Check sheet for the modelled part. Datum: model origin and axes. Units: mm. A direction names the side the tool comes from. Give positions to 0.01 mm unless a question says otherwise; leave off trailing zeros. Write each loop counter-clockwise with the first axis right and the second up, starting at its lowest first coordinate (ties: lowest second). Pieces come first, ordered by that corner, then holes. Notation, with made-up numbers: M 45.25,-31 L 79.25,-31 A17 ccw 79.25,-17 Z; hole C 70,4 d11. An arc over 180 degrees is marked long. Write item = value, one per line. Start each with the question number.
1) Scan lines: L1, parallel to Y at x = 22, z = 0.7; L2, parallel to Z at x = -4, y = -5; L3, parallel to Y at x = 0, z = 1.3. Record each from-to range of solid material in increasing order.
2) Sectioned sample at C-C, the plane x = 19. Record the cut outline in (y, z).
3) Sectioned sample at B-B, the plane y = 1. Record the cut outline in (x, z).
4) Set-up check for faces 1 (the face through (-1.636, -13.625, 1.566)), 2 (the face through (-9, 12, 1)), 3 (the face through (-1.7, -15.9, 2.5)), 4 (the face through (23.8, -15.2, 2.5)), 5 (the face through (-2, 10, 3)): record each of +Z, -Z, +X, -X, +Y, -Y from which the full face is reachable in a straight line by a thin tool's end or side.
5) Sectioned sample at D-D, the plane z = 1.5. Record the cut outline in (x, y), then the cut area to 3 significant figures.
6) Sectioned sample at A-A, the plane x = 0. Record the cut outline in (y, z).
7) Gauge pin test, flat ends, axial feed: pin 1 (0.5 mm diameter, centred on y = 1.5, z = 1.5, fed in from -X); pin 2 (4 mm diameter, centred on x = 19, y = -10, fed in from +Z); pin 3 (0.5 mm diameter, centred on x = -7.5, z = 2.5, fed in from -Y). Record the tip position at first contact, or that the pin passes through.
Autodesk Inventor part; units mm, degrees
ref_plane "YZ Plane" through (0, 0, 0) normal (1, 0, 0) x (0, 1, 0)
ref_plane "XZ Plane" through (0, 0, 0) normal (0, 1, 0) x (-1, 0, 0)
ref_plane "XY Plane" through (0, 0, 0) normal (0, 0, 1) x (1, 0, 0)
sketch "Sketch1" plane through (0, 0, 0) normal (0, 0, 1) x (1, 0, 0)
  line L0 (-28, 16.5) -> (28, 16.5)
  line L1 (28, 16.5) -> (28, -16.5)
  line L2 (28, -16.5) -> (-28, -16.5)
  line L3 (-28, -16.5) -> (-28, 16.5)
  point P0 (0, 0)
  dimension "d0" = 33
  dimension "d1" = 56
  dimension "d2" = 16.5
  dimension "d3" = 28
extrude "Extrusion1" add sketch "Sketch1" along normal blind 2
sketch "Sketch2" plane through (0, 0, 2) normal (0, 0, 1) x (1, 0, 0)
  line L0 (-28, 16.5) -> (-28, -16.5)
  line L1 (-28, -16.5) -> (28, -16.5)
  circle A0 centre (0, 13.5) radius 1
  circle A1 centre (22, 13.5) radius 1
  point P0 (0, 0)
  dimension "d6" = 28
  dimension "d7" = 30
  dimension "d8" = 50
  dimension "d9" = 30
  dimension "d10" = 2
  dimension "d11" = 2
extrude "Extrusion2" cut sketch "Sketch2" against normal blind 2
sketch "Sketch3" plane through (0, 0, 2) normal (0, 0, 1) x (1, 0, 0)
  line L0 (-28, 16.5) -> (-28, -16.5)
  line L1 (-28, 11.5) -> (24, 11.5)
  line L2 (24, 11.5) -> (24, -14.7)
  line L3 (24, -14.7) -> (-28, -14.7)
  line L4 (-28, -14.7) -> (-28, 11.5)
  line L5 (-28, -16.5) -> (28, -16.5)
  line L6 (-28, 11.5) -> (24, 11.5)
  line L7 (24, 11.5) -> (24, 9.1)
  line L8 (24, 9.1) -> (-28, 9.1)
  line L9 (-28, 9.1) -> (-28, 11.5)
  point P0 (0, 0)
  point P1 (-28, 9.1)
  point P2 (-28, -14.7)
  dimension "d14" = 1.8
  dimension "d15" = 28
  dimension "d16" = 2.4
  dimension "d17" = 52
extrude "Extrusion3" cut sketch "Sketch3" against normal blind 1 contours L8 L2 L3 L0
sketch "Sketch4" plane through (0, 0, 2) normal (0, 0, 1) x (1, 0, 0)
  line L0 (-28, -14.7) -> (-28, 9.1)
  line L1 (-28, -16.5) -> (28, -16.5)
  circle A0 centre (25.87, -14.63) radius 1
  point P0 (0, 0)
  point P1 (-28, -14.1)
  dimension "d23" = 53.87
  dimension "d24" = 1.87
  dimension "d25" = 2
extrude "Extrusion4" cut sketch "Sketch4" against normal blind 2
chamfer "Chamfer2" distance 3 angle 45 1 edges at (28, 16.5, 1)
sketch "Sketch8" plane through (0, 0, 2) normal (0, 0, 1) x (1, 0, 0)
  line L0 (25, 16.5) -> (-28, 16.5)
  line L1 (-28, 16.5) -> (-9, 16.5)
  line L2 (-9, 16.5) -> (-9, 10.3)
  line L3 (-9, 10.3) -> (-28, 10.3)
  line L4 (-28, 10.3) -> (-28, 16.5)
  line L5 (-28, 9.1) -> (24, 9.1)
  point P0 (0, 0)
  dimension "d40" = 19
  dimension "d41" = 1.2
extrude "Extrusion7" cut sketch "Sketch8" against normal blind 2
chamfer "Chamfer4" distance 3 angle 45 1 edges at (-9, 16.5, 1)
sketch "Sketch9" plane through (0, 0, 2) normal (0, 0, 1) x (1, 0, 0)
  line L0 (-28, 10.3) -> (-9, 10.3)
  line L1 (-28, 9.1) -> (24, 9.1)
  line L2 (-28, 10.3) -> (24, 10.3)
  line L3 (24, 10.3) -> (24, 9.1)
  line L4 (24, 9.1) -> (-28, 9.1)
  line L5 (-28, 9.1) -> (-28, 10.3)
  line L6 (24, -14.7) -> (-28, -14.7)
  line L7 (-28, -14.7) -> (24, -14.7)
  line L8 (24, -14.7) -> (24, -15.9)
  line L9 (24, -15.9) -> (-28, -15.9)
  line L10 (-28, -15.9) -> (-28, -14.7)
  line L11 (24, 9.1) -> (24, -14.7)
  point P0 (0, 0)
  dimension "d47" = 1.2
extrude "Extrusion8" add sketch "Sketch9" along normal blind 1
fillet "Fillet1" radius 3 2 edges at (-2, 9.1, 1) (-2, -14.7, 1)
sketch "Sketch10" plane through (0, 0, 3) normal (0, 0, 1) x (1, 0, 0)
  line L0 (24, 9.1) -> (24, 10.3)
  line L1 (-28, -15.9) -> (24, -15.9)
  line L2 (24, 10.3) -> (23.8, 10.3)
  line L3 (23.8, 10.3) -> (23.8, -15.9)
  line L4 (23.8, -15.9) -> (24, -15.9)
  line L5 (24, -15.9) -> (24, 10.3)
  point P0 (0, 0)
  dimension "d51" = 0.2
extrude "Extrusion9" cut sketch "Sketch10" against normal blind 1
properties part number "hdmi_base_plate"
Data:
q1.L1 = -16.5 to 12.5, 14.5 to 16.5
q1.L2 = 0 to 1
q1.L3 = -16.5 to -13.18, 7.58 to 12.5, 14.5 to 16.5
q2.outline = M -16.5,0 L 16.5,0 L 16.5,2 L 10.3,2 L 10.3,3 L 9.1,3 A3 cw 6.27,1 L -11.87,1 A3 cw -14.7,3 L -15.9,3 L -15.9,2 L -16.5,2 Z
q3.outline = M -28,0 L 28,0 L 28,2 L 24,2 L 24,1 L -28,1 Z
q4.face_1 = +Z, -X
q4.face_2 = +Z, -Z, -X, +Y
q4.face_3 = +Z, +X, -X, -Y
q4.face_4 = +Z, +X, +Y, -Y
q4.face_5 = +Z, +X, -X, +Y, -Y
q5.outline = M -28,-16.5 L 28,-16.5 L 28,13.5 L 25,16.5 L -6,16.5 L -9,13.5 L -9,10.3 L -28,10.3 L -28,7.93 L 24,7.93 L 24,-13.53 L -28,-13.53 Z; hole C 0,13.5 d2; hole C 22,13.5 d2; hole C 25.87,-14.63 d2
q5.area = 596 mm2
q6.outline = M -16.5,0 L 12.5,0 L 12.5,2 L 10.3,2 L 10.3,3 L 9.1,3 A3 cw 6.27,1 L -11.87,1 A3 cw -14.7,3 L -15.9,3 L -15.9,2 L -16.5,2 Z; M 14.5,0 L 16.5,0 L 16.5,2 L 14.5,2 Z
q7.pin_1 = 24
q7.pin_2 = 1
q7.pin_3 = -15.9
